Autodesk Inventor part; units mm, degrees
ref_plane "YZ Plane" through (0, 0, 0) normal (1, 0, 0) x (0, 1, 0)
ref_plane "XZ Plane" through (0, 0, 0) normal (0, 1, 0) x (-1, 0, 0)
ref_plane "XY Plane" through (0, 0, 0) normal (0, 0, 1) x (1, 0, 0)
sketch "Sketch1" plane through (0, 0, 0) normal (0, 1, 0) x (-1, 0, 0)
  line L0 (0, 0) -> (-17.78, 0)
  line L1 (-17.78, 0) -> (-17.78, -16.764)
  line L2 (-17.78, -16.764) -> (0, -16.764)
  line L3 (0, -16.764) -> (0, 0)
  dimension "d0" = 17.78
  dimension "d1" = 16.764
extrude "Extrusion1" add sketch "Sketch1" along normal blind 2.54
sketch "Sketch2" plane through (0, 2.54, 0) normal (0, 1, 0) x (1, 0, 0)
  line L0 (0, 0) -> (17.78, 0)
  line L1 (0, 0) -> (3.81, 0)
  line L2 (3.81, 0) -> (3.81, 3.81)
  line L3 (3.81, 3.81) -> (0, 3.81)
  line L4 (0, 3.81) -> (0, 0)
  line L5 (17.78, 16.764) -> (0, 16.764)
  line L6 (0, 16.764) -> (3.81, 16.764)
  line L7 (3.81, 16.764) -> (3.81, 12.954)
  line L8 (3.81, 12.954) -> (0, 12.954)
  line L9 (0, 12.954) -> (0, 16.764)
  line L10 (17.7651, 0) -> (13.9551, 0)
  line L11 (13.9551, 0) -> (13.9551, 3.81)
  line L12 (13.9551, 3.81) -> (17.7651, 3.81)
  line L13 (17.7651, 3.81) -> (17.7651, 0)
  line L14 (17.78, 0) -> (17.78, 16.764)
  line L15 (17.78, 16.764) -> (13.97, 16.764)
  line L16 (13.97, 16.764) -> (13.97, 12.954)
  line L17 (13.97, 12.954) -> (17.78, 12.954)
  line L18 (17.78, 12.954) -> (17.78, 16.764)
  point P0 (1.905, 1.905)
  point P1 (15.875, 1.905)
  point P2 (15.875, 14.859)
  point P3 (1.905, 14.859)
  dimension "d4" = 3.81
  dimension "d5" = 3.81
  dimension "d6" = 3.81
  dimension "d7" = 3.81
  dimension "d8" = 3.81
  dimension "d9" = 3.81
  dimension "d10" = 3.81
  dimension "d11" = 3.81
hole "Hole1" at (1.905, 2.54, -1.905) at (15.875, 2.54, -1.905) at (15.875, 2.54, -14.859) at (1.905, 2.54, -14.859) direction (0, -1, 0) diameter 3.048 depth 10.16 tip angle 118
properties part number "Phone Mount Cover V1"
Can you work these out from the model? Positions are in its coordinate system, mm. Give positions to 0.01 mm unless a question says otherwise; leave off trailing zeros. Write each loop counter-clockwise with the first axis right and the second up, starting at its lowest first coordinate (ties: lowest second). Pieces come first, ordered by that corner, then holes. Notation, with made-up numbers: (82, 8) - (89, 8) arc R11 cw to (89, 23) - close; hole circle Ø6 at (27.25, 23.5). An arc over 180 degrees is marked (long way). Write item = value, one per line. Start each with the question number.
1. Please list where these lines run through material, in increasing order: line 1 (X direction, y = 1.7, z = -14.75); line 2 (Z direction, x = 15.75, y = 0.45); line 3 (X direction, y = 0.25, z = -2.75).
2. Imagine slicing it at A-A (x = 15.25). Please give me the cut outline in (y, z).
3. Thinking about a two-plate mould opening in Z: for faces 1 (the face through (9, 1, -16.764)), 2 (the face through (14.364, 1.252, -2.103)), 3 (the face through (0, 1, -8)), which applies, released by +Z, released by -Z, zero draft, split by the parting line, or undercut?
4. For pin 1 (2.5 mm diameter, centred on x = 15.875, z = -1.905, fed in from +Y), with a flat end and sliding along its axis, tell me the tip position at first contact or that it passes through.
5. Imagine slicing it at B-B (z = -14.5). Please give me the cut outline in (x, y), and give its area (3 significant figures).
6. Imagine slicing it at C-C (y = 0.7). Please give me the cut outline in (x, z) (3 decimals), and give its area (3 significant figures).
Worked answers:
q1.line_1 = 0 to 0.38, 3.43 to 14.35, 17.4 to 17.78
q1.line_2 = -16.76 to -16.38, -13.34 to -3.42, -0.39 to 0
q1.line_3 = 0 to 0.64, 3.17 to 14.61, 17.14 to 17.78
q2.outline = (0, -16.76) - (2.54, -16.76) - (2.54, -16.25) - (0, -16.25) - close; (0, -13.47) - (2.54, -13.47) - (2.54, -3.29) - (0, -3.29) - close; (0, -0.52) - (2.54, -0.52) - (2.54, 0) - (0, 0) - close
q3.face_1 = released by -Z
q3.face_2 = undercut
q3.face_3 = zero draft
q4.pin_1 = through
q5.outline = (0, 0) - (0.42, 0) - (0.42, 2.54) - (0, 2.54) - close; (3.39, 0) - (14.39, 0) - (14.39, 2.54) - (3.39, 2.54) - close; (17.36, 0) - (17.78, 0) - (17.78, 2.54) - (17.36, 2.54) - close
q5.area = 30.1 mm2
q6.outline = (0, -16.764) - (17.78, -16.764) - (17.78, 0) - (0, 0) - close; hole circle Ø3.048 at (1.905, -14.859); hole circle Ø3.048 at (1.905, -1.905); hole circle Ø3.048 at (15.875, -14.859); hole circle Ø3.048 at (15.875, -1.905)
q6.area = 269 mm2
